The drawing under review shows one solid part. Ordinate dimensions are in mm from its lowest x, y, z. A direction names the side the tool comes from. Round coordinates to 2 decimals unless told otherwise and drop trailing zeros. Write each loop counter-clockwise with the first axis right and the second up, starting at its lowest first coordinate (ties: lowest second). Pieces come first, ordered by that corner, then holes. Notation, with made-up numbers: (17.25, 89) -> (55.25, 89) arc R16 cw to (55.25, 97) -> close; hole circle Ø10 at (10, 60). An arc over 180 degrees is marked (long way). Answer in a Markdown table with one row per item.
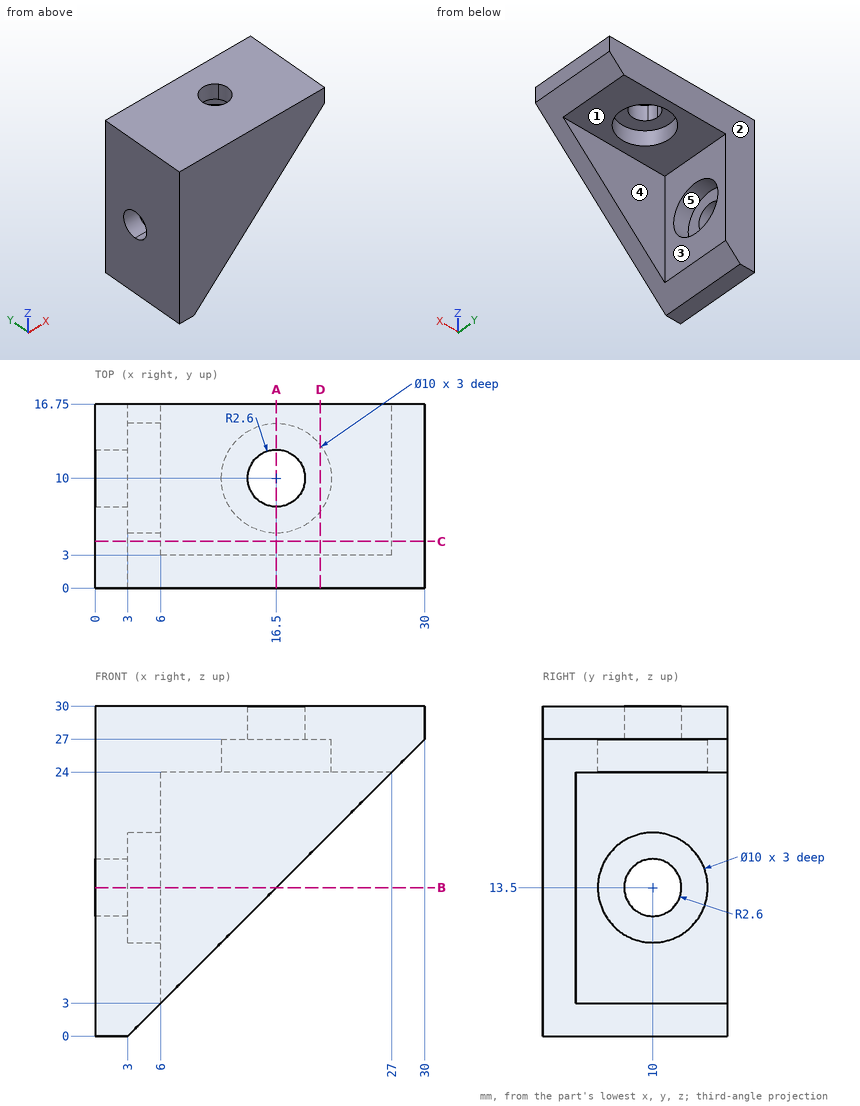
1) Mouldability with a two-part tool opening along Y and no side actions: class the marked faces 3, 4 and 5 as pulls with the +Y half, pulls with the -Y half, needs draft (parallel to the pull), parting line crosses it, or undercut.
Solved:
| item | result |
|---|---|
| face 3 | needs draft |
| face 4 | pulls with the +Y half |
| face 5 | undercut |
2) Consider section D-D on x = 20.5. State the section outline as (y, z) points, then the cut area to 3 significant figures.
Solved:
| item | result |
|---|---|
| outline | (0, 17.5) -> (3, 17.5) -> (3, 24) -> (7, 24) -> (7, 27) -> (13, 27) -> (13, 24) -> (16.75, 24) -> (16.75, 30) -> (0, 30) -> close |
| area | 102 mm² |
3) For the marked faces 1 and 2, list the 3-axis set-ups (+Z, -Z, +X, -X, +Y, -Y) from which the entire face can be reached by the end or side of a thin tool; tool diameter is ignored.
Solved:
| item | result |
|---|---|
| face 1 | -Z, +X, +Y |
| face 2 | +Z, -Z, +X, -X, +Y |
4) Consider section A-A on x = 16.5. State the section outline as (y, z) points, then the cut area to 3 significant figures.
Solved:
| item | result |
|---|---|
| outline | (0, 13.5) -> (3, 13.5) -> (3, 24) -> (5, 24) -> (5, 27) -> (7.4, 27) -> (7.4, 30) -> (0, 30) -> close; (12.6, 27) -> (15, 27) -> (15, 24) -> (16.75, 24) -> (16.75, 30) -> (12.6, 30) -> close |
| area | 86.4 mm² |
5) Consider section B-B on z = 13.5. State the section outline as (x, y) points.
Solved:
| item | result |
|---|---|
| outline | (0, 0) -> (16.5, 0) -> (16.5, 3) -> (6, 3) -> (6, 5) -> (3, 5) -> (3, 7.4) -> (0, 7.4) -> close; (0, 12.6) -> (3, 12.6) -> (3, 15) -> (6, 15) -> (6, 16.75) -> (0, 16.75) -> close |
6) Consider section C-C on y = 4.25. State the section outline as (x, z) points.
Solved:
| item | result |
|---|---|
| outline | (0, 0) -> (3, 0) -> (6, 3) -> (6, 24) -> (27, 24) -> (30, 27) -> (30, 30) -> (0, 30) -> close |
7) Clearance check with flat-ended pins moving along their axes: pin 1 Ø8 at (y, z) = (9.5, 14) entering from +X; pin 2 Ø10 at (x, z) = (27, 18.5) entering from +Y; pin 3 Ø4 at (y, z) = (9, 16.5) entering from +X; pin 4 Ø12 at (x, z) = (26, 11) entering from -Y. State where each tip first meets the part, or that it passes through.
Solved:
| item | result |
|---|---|
| pin 1 | x = 3 |
| pin 2 | y = 3 |
| pin 3 | x = 6 |
| pin 4 | through |
8) For line 1 (Y direction, x = 16.5, z = 24.75); line 2 (Y direction, x = 11.5, z = 18.75); line 3 (X direction, y = 8, z = 19.75), list the stretches that pass through material, from the lowest coordinate up. Write a range as [from, to].
Solved:
| item | result |
|---|---|
| line 1 | [0, 5], [15, 16.75] |
| line 2 | [0, 3] |
| line 3 | [0, 6] |
